Here's the drawing with two shaded views (mm, measured from the low corner). I have some questions. A direction names the side the tool comes from. Coordinates: 2 decimals unless noted, no trailing zeros. Loops run counter-clockwise (first coordinate to the right, second up) from the corner with the lowest first, then second, coordinate; pieces in that order, holes last. Notation, with made-up numbers: (64, -1) - (99, -1) arc R26 ccw to (99, 25) - close; hole circle Ø5 at (-21, 9). An arc over 180 degrees is marked (long way). Use a Markdown table: item, result.
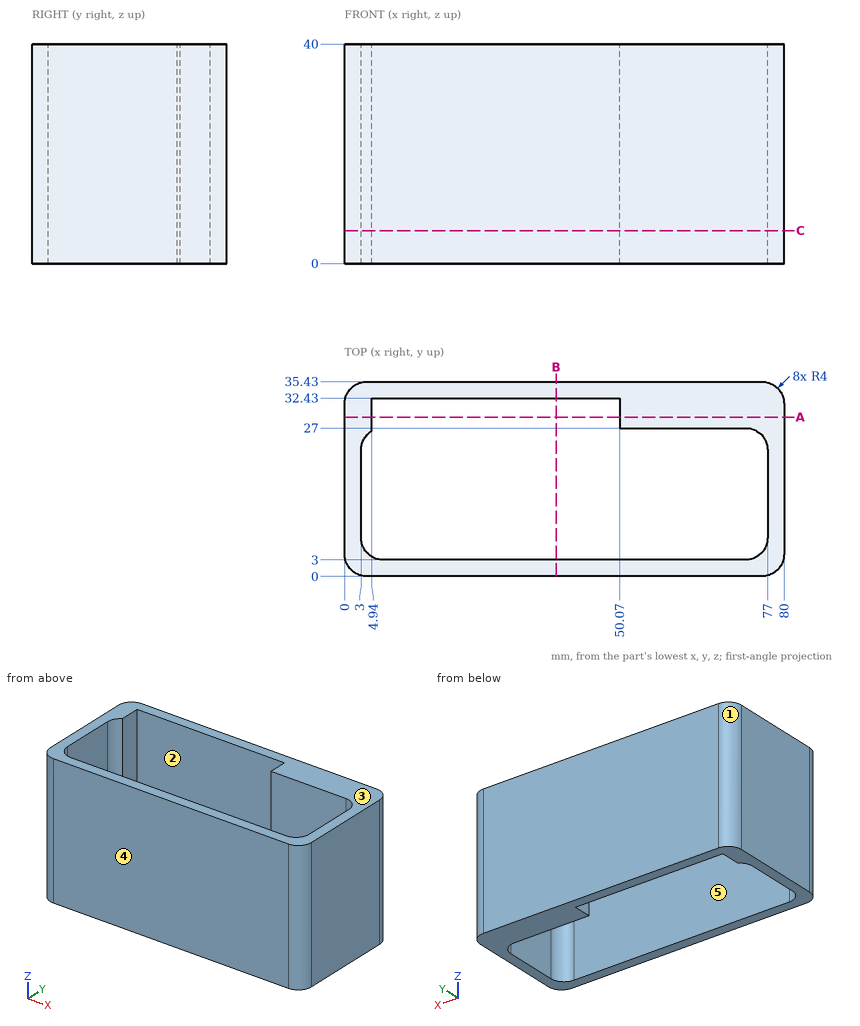
Q1. I want a section at C-C, the plane z = 6. Write out the boundary of the cut face in (x, y), then the cut area to 3 significant figures.
Check values:
| item | result |
|---|---|
| outline | (0, 4) arc R4 ccw to (4, 0) - (76, 0) arc R4 ccw to (80, 4) - (80, 31.43) arc R4 ccw to (76, 35.43) - (4, 35.43) arc R4 ccw to (0, 31.43) - close; hole (3, 7) arc R4 ccw to (7, 3) - (73, 3) arc R4 ccw to (77, 7) - (77, 23) arc R4 ccw to (73, 27) - (50.07, 27) - (50.07, 32.43) - (4.94, 32.43) - (4.94, 26.43) arc R4 ccw to (3, 23) - close |
| area | 813 mm^2 |
Q2. I want a section at B-B, the plane x = 38.5. Write out the boundary of the cut face in (y, z), then the cut area to 3 significant figures.
Check values:
| item | result |
|---|---|
| outline | (0, 0) - (3, 0) - (3, 40) - (0, 40) - close; (32.43, 0) - (35.43, 0) - (35.43, 40) - (32.43, 40) - close |
| area | 240 mm^2 |
Q3. Will this pin go through, and if not, where does the flat tip stop? P1, Ø8, axis at x = 12, y = 9, coming from the -Z side.
Check values:
| item | result |
|---|---|
| P1 | through |
Q4. If we mould it in two halves opening along Y, with no side actions, what happens to the marked faces 3, 4 and 5? For each: pulls with the +Y half, pulls with the -Y half, needs draft (parallel to the pull), parting line crosses it, or undercut.
Check values:
| item | result |
|---|---|
| face 3 | needs draft |
| face 4 | pulls with the -Y half |
| face 5 | undercut |
Q5. Please list where these lines run through material, in increasing order: L1, parallel to Y at x = 16, z = 16.5; L2, parallel to X at y = 28, z = 12.5; L3, parallel to Y at x = 71, z = 22.5. Write a range as from..to.
Check values:
| item | result |
|---|---|
| L1 | 0..3, 32.43..35.43 |
| L2 | 0..4.94, 50.07..80 |
| L3 | 0..3, 27..35.43 |
Q6. Which directions (+Z, -Z, +X, -X, +Y, -Y) give clear straight access to the entire face, cutting with the end or side of a thin tool? Please do the marked faces 1 and 2.
Check values:
| item | result |
|---|---|
| face 1 | +Z, -Z, -X, +Y |
| face 2 | +Z, -Z |
Q7. I want a section at A-A, the plane y = 29. Write out the boundary of the cut face in (x, z).
Check values:
| item | result |
|---|---|
| outline | (0, 0) - (4.94, 0) - (4.94, 40) - (0, 40) - close; (50.07, 0) - (80, 0) - (80, 40) - (50.07, 40) - close |
